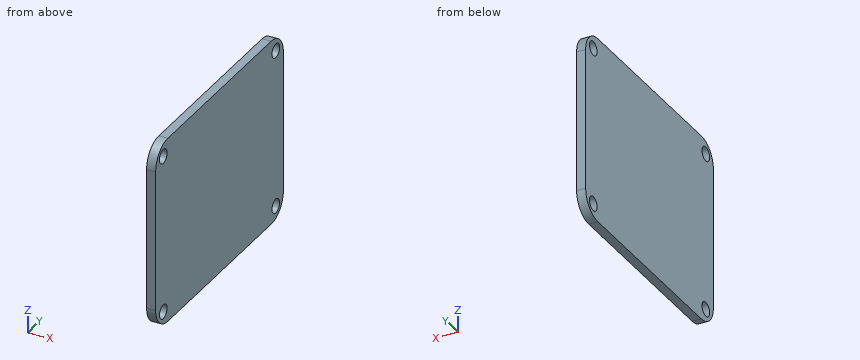
```python
from build123d import *

# Parameters (mm, degrees)
SKETCH2_R           = 1.25
BOSS_EXTRUDE1_DEPTH = 1.6


with BuildPart() as part:
    # Sketch2 → Boss-Extrude1 (new body)
    with BuildSketch(Plane.YZ):
        with BuildLine():
            Line((-17, -16.5), (17, -16.5))
            ThreePointArc((17, -16.5), (19.828427125, -15.328427125), (21, -12.5))
            Line((21, -12.5), (21, 12.5))
            ThreePointArc((21, 12.5), (19.828427125, 15.328427125), (17, 16.5))
            Line((17, 16.5), (-17, 16.5))
            ThreePointArc((-17, 16.5), (-19.828427125, 15.328427125), (-21, 12.5))
            Line((-21, 12.5), (-21, -12.5))
            ThreePointArc((-21, -12.5), (-19.828427125, -15.328427125), (-17, -16.5))
        make_face()
        with Locations(Location((-18.5, 14, 0), (0, 0, 270))):
            Circle(SKETCH2_R, mode=Mode.SUBTRACT)
        with Locations(Location((-18.5, -14, 0), (0, 0, 270))):
            Circle(SKETCH2_R, mode=Mode.SUBTRACT)
        with Locations(Location((18.5, 14, 0), (0, 0, 270))):
            Circle(SKETCH2_R, mode=Mode.SUBTRACT)
        with Locations(Location((18.5, -14, 0), (0, 0, 270))):
            Circle(SKETCH2_R, mode=Mode.SUBTRACT)
    extrude(amount=BOSS_EXTRUDE1_DEPTH)


solid = part.part
```
Source: CAD feature listing. Evaluate the final solid. Frame: model axes, mm. Give positions to 0.01 mm unless a question says otherwise; leave off trailing zeros. Order: outer loops, then holes, each group sorted by start corner. A loop starts at its lowest first (then second) coordinate and runs counter-clockwise, first axis right, second up. Notation, with made-up numbers: (16, -30.5) -> (65, -30.5) arc R29 cw to (65, -0.5) -> close; hole circle Ø11 at (-37.5, -17). An arc over 180 degrees is marked (long way). Use a Markdown table: item, result.
Q1. Section C-C (y = -18.5). Return the cut outline in (x, z), and give its area (3 significant figures).
A:
| item | result |
|---|---|
| outline | (0, -16.21) -> (1.6, -16.21) -> (1.6, -15.25) -> (0, -15.25) -> close; (0, -12.75) -> (1.6, -12.75) -> (1.6, 12.75) -> (0, 12.75) -> close; (0, 15.25) -> (1.6, 15.25) -> (1.6, 16.21) -> (0, 16.21) -> close |
| area | 43.9 mm^2 |
Q2. Material intervals for line 1 (Y direction, x = 0.9, z = 14); line 2 (Y direction, x = 0.95, z = 13.5), sorted ascending. Write a range as [from, to].
A:
| item | result |
|---|---|
| line 1 | [-20.71, -19.75], [-17.25, 17.25], [19.75, 20.71] |
| line 2 | [-20.87, -19.65], [-17.35, 17.35], [19.65, 20.87] |
Q3. Section A-A (z = 14). Return the cut outline in (x, y).
A:
| item | result |
|---|---|
| outline | (0, -20.71) -> (1.6, -20.71) -> (1.6, -19.75) -> (0, -19.75) -> close; (0, -17.25) -> (1.6, -17.25) -> (1.6, 17.25) -> (0, 17.25) -> close; (0, 19.75) -> (1.6, 19.75) -> (1.6, 20.71) -> (0, 20.71) -> close |
Q4. First-contact query: P1, Ø1, axis at y = 14, z = 8.5, coming from the -X side. Flat tip, straight axial feed; report the tip coordinate or a pass-through.
A:
| item | result |
|---|---|
| P1 | x = 0 |
Q5. Section B-B (x = 1.25). Return the cut outline in (y, z).
A:
| item | result |
|---|---|
| outline | (-21, -12.5) arc R4 ccw to (-17, -16.5) -> (17, -16.5) arc R4 ccw to (21, -12.5) -> (21, 12.5) arc R4 ccw to (17, 16.5) -> (-17, 16.5) arc R4 ccw to (-21, 12.5) -> close; hole circle Ø2.5 at (-18.5, -14); hole circle Ø2.5 at (-18.5, 14); hole circle Ø2.5 at (18.5, -14); hole circle Ø2.5 at (18.5, 14) |
